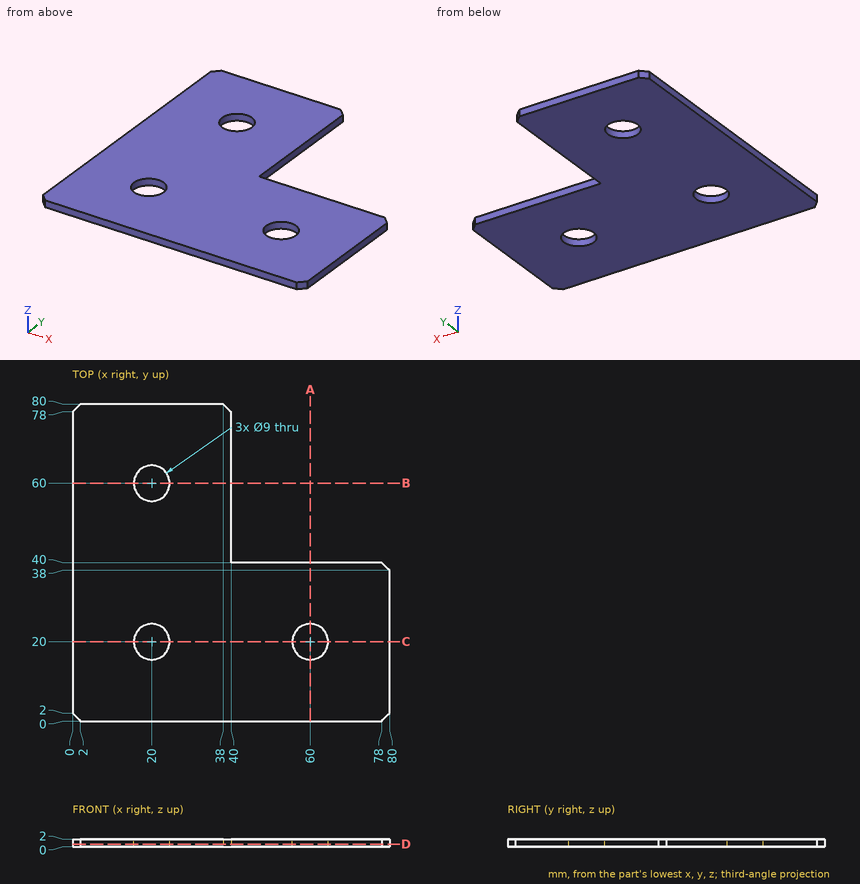
Geometry: see drawing. Coordinates: mm, zero at the bounding-box minimum. Give positions to 0.01 mm unless a question says otherwise; leave off trailing zeros. Loops run counter-clockwise (first coordinate to the right, second up) from the corner with the lowest first, then second, coordinate; pieces in that order, holes last. Notation, with made-up numbers: M 80.5,32.25 L 99.5,32.25 A15 ccw 99.5,44.25 Z; hole C 78.5,19 d11. An arc over 180 degrees is marked long. Use one line per item in the form item = value.
1. Section query A-A, the plane x = 60. Return the cut outline in (y, z).
Numbers:
outline = M 0,0 L 15.5,0 L 15.5,2 L 0,2 Z; M 24.5,0 L 40,0 L 40,2 L 24.5,2 Z
2. Section query D-D, the plane z = 0.7. Return the cut outline in (x, y).
Numbers:
outline = M 0,2 L 2,0 L 78,0 L 80,2 L 80,38 L 78,40 L 40,40 L 40,78 L 38,80 L 2,80 L 0,78 Z; hole C 20,20 d9; hole C 20,60 d9; hole C 60,20 d9
3. Section query C-C, the plane y = 20. Return the cut outline in (x, z), and give its area (3 significant figures).
Numbers:
outline = M 0,0 L 15.5,0 L 15.5,2 L 0,2 Z; M 24.5,0 L 55.5,0 L 55.5,2 L 24.5,2 Z; M 64.5,0 L 80,0 L 80,2 L 64.5,2 Z
area = 124 mm²
4. Line query: L1, parallel to Y at x = 20, z = 0.65; L2, parallel to Y at x = 60, z = 1.4. Output: solid intervals per line, ascending.
Numbers:
L1 = 0 to 15.5, 24.5 to 55.5, 64.5 to 80
L2 = 0 to 15.5, 24.5 to 40
